```python
from build123d import *

# Parameters (mm, degrees)
SKETCH3_W           = 11.5
SKETCH3_H           = 9.994310106
SKETCH3_R           = 1.5
BOSS_EXTRUDE2_DEPTH = 13.7


with BuildPart() as part:
    # Sketch3 → Boss-Extrude2 (new body)
    with BuildSketch(Plane.XY):
        Rectangle(SKETCH3_W, SKETCH3_H)
        with Locations(Location((3.662514997, 0, 0), (0, 0, 180))):
            Circle(SKETCH3_R, mode=Mode.SUBTRACT)
        with Locations(Location((-3.662514997, 0, 0), (0, 0, 180))):
            Circle(SKETCH3_R, mode=Mode.SUBTRACT)
    extrude(amount=BOSS_EXTRUDE2_DEPTH)


solid = part.part
```
Geometry check sheet. Reference: the model listing, model coordinates, mm. Round coordinates to 2 decimals unless told otherwise and drop trailing zeros. Order: outer loops, then holes, each group sorted by start corner. A loop starts at its lowest first (then second) coordinate and runs counter-clockwise, first axis right, second up. Notation, with made-up numbers: (32, 1) - (62, 1) arc R24 ccw to (62, 21) - close; hole circle Ø10 at (-31, 50.25). An arc over 180 degrees is marked (long way). Use a Markdown table: item, result. Add a question column.
1) Mould release check, pull along Y, two halves, no side actions. Record for faces 1 (the flat face through (0, 0, 13.7)), 2 (the flat face through (0, -4.997, 7)), 3 (the cylindrical face through (2.23, -0.45, 6.75)), 4 (the flat face through (0, 4.997, 7)): released by +Y, released by -Y, zero draft, split by the parting line, or undercut.
2) Section check A-A (y = 0). Record the cut outline in (x, z), then the cut area to 4 significant figures.
3) Section check B-B (x = -4). Record the cut outline in (y, z).
4) Thickness scan on line 1 along X through (y, z) = (-1.25, 7); line 2 along Y through (x, z) = (3.75, 7.25); line 3 along X through (y, z) = (0.75, 2.75). Record the ranges inside material, lowest first.
5) Section check C-C (z = 10). Record the cut outline in (x, y), then the cut area to 3 significant figures.
Established:
| question | item | result |
|---|---|---|
| 1 | face 1 | zero draft |
| 1 | face 2 | released by -Y |
| 1 | face 3 | undercut |
| 1 | face 4 | released by +Y |
| 2 | outline | (-5.75, 0) - (-5.16, 0) - (-5.16, 13.7) - (-5.75, 13.7) - close; (-2.16, 0) - (2.16, 0) - (2.16, 13.7) - (-2.16, 13.7) - close; (5.16, 0) - (5.75, 0) - (5.75, 13.7) - (5.16, 13.7) - close |
| 2 | area | 75.35 mm2 |
| 3 | outline | (-5, 0) - (-1.46, 0) - (-1.46, 13.7) - (-5, 13.7) - close; (1.46, 0) - (5, 0) - (5, 13.7) - (1.46, 13.7) - close |
| 4 | line 1 | -5.75 to -4.49, -2.83 to 2.83, 4.49 to 5.75 |
| 4 | line 2 | -5 to -1.5, 1.5 to 5 |
| 4 | line 3 | -5.75 to -4.96, -2.36 to 2.36, 4.96 to 5.75 |
| 5 | outline | (-5.75, -5) - (5.75, -5) - (5.75, 5) - (-5.75, 5) - close; hole circle Ø3 at (-3.66, 0); hole circle Ø3 at (3.66, 0) |
| 5 | area | 101 mm2 |
